Verification items for the finished model (mm, model axes). Face numbers are marked on the shaded views. Give positions to 0.01 mm unless a question says otherwise; leave off trailing zeros. Loops run counter-clockwise (first coordinate to the right, second up) from the corner with the lowest first, then second, coordinate; pieces in that order, holes last. Notation, with made-up numbers: M 58,33 L 84,33 A19 cw 84,68 Z; hole C 27.5,-8 d8. An arc over 180 degrees is marked long. Put each result on its own line as item: value. Start each with the question number.
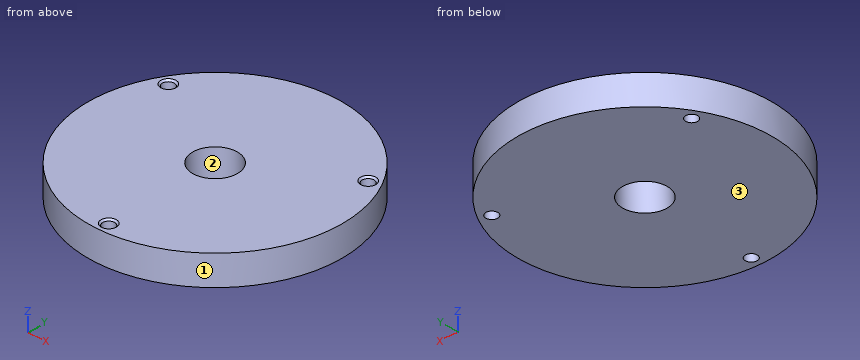
from build123d import *

# Parameters (mm, degrees)
SKETCH1_R                       = 17
BOSS_EXTRUDE1_DEPTH             = 4
M2X0_4_TAPPED_HOLE1_D           = 1.6
M2X0_4_TAPPED_HOLE1_CSINK_D     = 2.05
M2X0_4_TAPPED_HOLE1_CSINK_ANGLE = 90
CIRPATTERN1_COUNT               = 3
SKETCH4_R                       = 3
CUT_EXTRUDE1_DEPTH              = 5


with BuildPart() as part:
    # Sketch1 → Boss-Extrude1 (new body)
    with BuildSketch(Plane.XY):
        Circle(SKETCH1_R)
    extrude(amount=-BOSS_EXTRUDE1_DEPTH)

    # M2x0.4 Tapped Hole1 (through all)
    with Locations(Plane.XY):
        with Locations((0, -15.5)):
            m2x0_4_tapped_hole1 = CounterSinkHole(M2X0_4_TAPPED_HOLE1_D / 2, M2X0_4_TAPPED_HOLE1_CSINK_D / 2, counter_sink_angle=M2X0_4_TAPPED_HOLE1_CSINK_ANGLE)

    # CirPattern1: M2x0.4 Tapped Hole1 ×3 about axis
    cirpattern1_axis = Axis((0, 0, 0), (0, 0, 1))
    for i in range(1, CIRPATTERN1_COUNT):
        add(m2x0_4_tapped_hole1.rotate(cirpattern1_axis, i * 360 / CIRPATTERN1_COUNT), mode=Mode.SUBTRACT)

    # Sketch4 → Cut-Extrude1 (cut, through all)
    with BuildSketch(Plane.XY):
        Circle(SKETCH4_R)
    extrude(amount=-CUT_EXTRUDE1_DEPTH, mode=Mode.SUBTRACT)


solid = part.part
Q1. Cross-section at D-D, the plane z = -2.35. Record the boundary of the cut face in (x, y), then the cut area to 3 significant figures.
Q2. Release check for a two-part mould opening along X. For the marked faces 1, 2 and 3 record: pulls with the +X half, pulls with the -X half, needs draft (parallel to the pull), parting line crosses it, or undercut.
Q3. Cross-section at B-B, the plane y = 0. Record the boundary of the cut face in (x, z), then the cut area to 3 significant figures.
Q4. Scan lines: L1, parallel to Y at x = 0, z = -1.35; L2, parallel to X at y = 7.5, z = -2.85; L3, parallel to X at y = -0.5, z = -0.85. Record each from-to range of solid material in increasing order.
Q5. Go/stop test with flat-tipped pins: pin 1 (1 mm diameter, centred on x = 0, y = -15.5, fed in from -Z) (3 decimals); pin 2 (2 mm diameter, centred on x = 10.5, z = -3.5, fed in from +Y); pin 3 (5 mm diameter, centred on x = 0.5, y = 3.5, fed in from +Z); pin 4 (1.8 mm diameter, centred on x = 13.42, y = 7.75, fed in from +Z). Record where each tip stops, or that it passes through.
Q6. Cross-section at A-A, the plane x = 0. Record the boundary of the cut face in (y, z) (3 decimals).
Q7. Cross-section at C-C, the plane y = 7.75. Record the boundary of the cut face in (x, z) (3 decimals), then the cut area to 3 significant figures.
Ans:
1. outline: C 0,0 d34; hole C -13.42,7.75 d1.6; hole C 0,0 d6; hole C 0,-15.5 d1.6; hole C 13.42,7.75 d1.6
1. area: 874 mm^2
2. face 1: parting line crosses it
2. face 2: undercut
2. face 3: needs draft
3. outline: M -17,-4 L -3,-4 L -3,0 L -17,0 Z; M 3,-4 L 17,-4 L 17,0 L 3,0 Z
3. area: 112 mm^2
4. L1: y = -17 to -16.3, -14.7 to -3, 3 to 17
4. L2: x = -15.26 to -14.18, -12.66 to 12.66, 14.18 to 15.26
4. L3: x = -16.99 to -2.96, 2.96 to 16.99
5. pin 1: passes through
5. pin 2: stops at y = 14.1
5. pin 3: stops at z = 0
5. pin 4: stops at z = -0.12
6. outline: M -17,-4 L -16.3,-4 L -16.3,-0.225 L -16.525,0 L -17,0 Z; M -14.7,-4 L -3,-4 L -3,0 L -14.475,0 L -14.7,-0.225 Z; M 3,-4 L 17,-4 L 17,0 L 3,0 Z
7. outline: M -15.131,-4 L -14.223,-4 L -14.223,-0.225 L -14.448,0 L -15.131,0 Z; M -12.623,-4 L 12.623,-4 L 12.623,-0.225 L 12.398,0 L -12.398,0 L -12.623,-0.225 Z; M 14.223,-4 L 15.131,-4 L 15.131,0 L 14.448,0 L 14.223,-0.225 Z
7. area: 108 mm^2
